Input: part model. Units: mm. Frame: model coordinates. Face numbers are marked on the shaded views. Round coordinates to 2 decimals unless told otherwise and drop trailing zeros. Loops run counter-clockwise (first coordinate to the right, second up) from the corner with the lowest first, then second, coordinate; pieces in that order, holes last. Notation, with made-up numbers: (53.5, 15) - (70.5, 15) arc R18 cw to (70.5, 39) - close; hole circle Ø1 at (72, -12.75). An arc over 180 degrees is marked (long way). Use CSV: the item, a comma, the result in double quotes. Start each with the question number.
1. Cut plane D-D (x = -1). Return loops of the section in (y, z).
2. Cut plane A-A (z = 0). Return loops of the section in (x, y) (3 decimals), and give its area (3 significant figures).
3. Cut plane C-C (y = 6.75). Return loops of the section in (x, z) (3 decimals).
4. Pull-direction query (Z, two-part tool) for the marked faces 1, 2 and 3; classes: +Z half, -Z half, draft (parallel to the pull), parting line (faces both ways), or undercut.
5. Pin query (flat end, axial travel): P1, Ø2, axis at y = 6, z = 18.5, coming from the +X side; P2, Ø2, axis at y = 10, z = 5, coming from the -X side; P3, Ø1.5, axis at y = 3, z = -17.5, coming from the +X side; P4, Ø7, axis at x = 0, z = 0, coming from the -Y side. Return the tip coordinate at first contact, or that it passes through.
6. Cut plane B-B (x = -15). Return loops of the section in (y, z).
7. Material intervals for probe 1 along X at (y, z) = (7.5, 0) (3 decimals); probe 2 along Y at (x, z) = (21, -21.5); probe 3 along X at (y, z) = (3.75, 15), sorted ascending. Write a range as from..to.
```python
from build123d import *

# Parameters (mm, degrees)
SKETCH_1_R          = 30.5
SKETCH_1_R_2        = 4
SKETCH_1_R_3        = 2
EXTRUDE_1_DEPTH     = 15
CUT_EXTRUDE_START   = 2
SKETCH_2_R          = 30.5
SKETCH_2_R_2        = 28.265
CUT_EXTRUDE_1_DEPTH = 11


with BuildPart() as part:
    # 草图1 → 凸台-拉伸1 (new body)
    with BuildSketch(Plane(origin=(0, 0, 0), x_dir=(1, 0, 0), z_dir=(0, 1, 0))):
        with Locations(Location((0, 0, 0), (0, 0, 270))):
            Circle(SKETCH_1_R)
        with Locations(Location((0, 0, 0), (0, 0, 270))):
            Circle(SKETCH_1_R_2, mode=Mode.SUBTRACT)
        with Locations(Location((0, 15, 0), (0, 0, 270))):
            Circle(SKETCH_1_R_3, mode=Mode.SUBTRACT)
        with Locations(Location((15, 0, 0), (0, 0, 270))):
            Circle(SKETCH_1_R_3, mode=Mode.SUBTRACT)
        with Locations(Location((0, -15, 0), (0, 0, 270))):
            Circle(SKETCH_1_R_3, mode=Mode.SUBTRACT)
        with Locations(Location((-15, 0, 0), (0, 0, 270))):
            Circle(SKETCH_1_R_3, mode=Mode.SUBTRACT)
    extrude(amount=EXTRUDE_1_DEPTH)

    # 草图2 → 切除-拉伸1 (cut)
    with BuildSketch(Plane(origin=(0, 0, 0), x_dir=(1, 0, 0), z_dir=(0, 1, 0)).offset(CUT_EXTRUDE_START)):
        with Locations(Location((0, 0, 0), (0, 0, 270))):
            Circle(SKETCH_2_R)
        with Locations(Location((0, 0, 0), (0, 0, 270))):
            Circle(SKETCH_2_R_2, mode=Mode.SUBTRACT)
    extrude(amount=CUT_EXTRUDE_1_DEPTH, mode=Mode.SUBTRACT)


solid = part.part
```
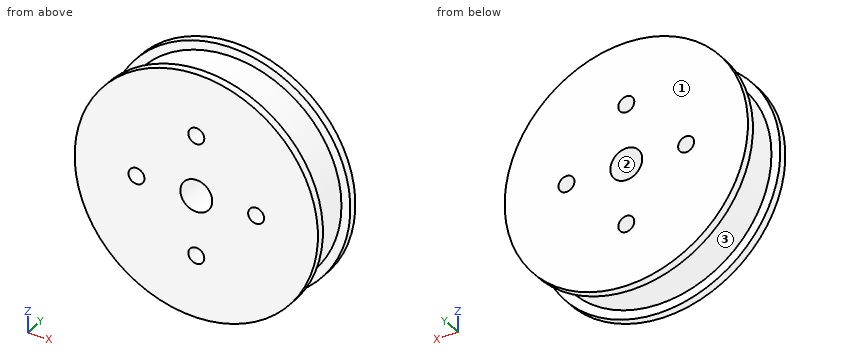
Established:
1,outline,"(0, -30.48) - (2, -30.48) - (2, -28.25) - (13, -28.25) - (13, -30.48) - (15, -30.48) - (15, -16.73) - (0, -16.73) - close; (0, -13.27) - (15, -13.27) - (15, -3.87) - (0, -3.87) - close; (0, 3.87) - (15, 3.87) - (15, 13.27) - (0, 13.27) - close; (0, 16.73) - (15, 16.73) - (15, 30.48) - (13, 30.48) - (13, 28.25) - (2, 28.25) - (2, 30.48) - (0, 30.48) - close"
2,outline,"(-30.5, 0) - (-17, 0) - (-17, 15) - (-30.5, 15) - (-30.5, 13) - (-28.265, 13) - (-28.265, 2) - (-30.5, 2) - close; (-13, 0) - (-4, 0) - (-4, 15) - (-13, 15) - close; (4, 0) - (13, 0) - (13, 15) - (4, 15) - close; (17, 0) - (30.5, 0) - (30.5, 2) - (28.265, 2) - (28.265, 13) - (30.5, 13) - (30.5, 15) - (17, 15) - close"
2,area,"626 mm2"
3,outline,"circle Ø56.53 at (0, 0); hole circle Ø4 at (-15, 0); hole circle Ø8 at (0, 0); hole circle Ø4 at (0, -15); hole circle Ø4 at (0, 15); hole circle Ø4 at (15, 0)"
4,face 1,"draft"
4,face 2,"undercut"
4,face 3,"parting line"
5,P1,"stops at x = 22.2"
5,P2,"stops at x = -27.98"
5,P3,"stops at x = 22.77"
5,P4,"passes through"
6,outline,"(0, -26.56) - (2, -26.56) - (2, -23.96) - (13, -23.96) - (13, -26.56) - (15, -26.56) - (15, -2) - (0, -2) - close; (0, 2) - (15, 2) - (15, 26.56) - (13, 26.56) - (13, 23.96) - (2, 23.96) - (2, 26.56) - (0, 26.56) - close"
7,probe 1,"x = -28.265..-17, -13..-4, 4..13, 17..28.265"
7,probe 2,"y = 0..2, 13..15"
7,probe 3,"x = -23.96..-2, 2..23.96"
